Read the model definition and answer for the solid it produces. Units are mm, in the model's axes. A direction names the side the tool comes from. Coordinates: 2 decimals unless noted, no trailing zeros. Write each loop counter-clockwise with the first axis right and the second up, starting at its lowest first coordinate (ties: lowest second). Pieces come first, ordered by that corner, then holes. Notation, with made-up numbers: (73.25, 30.5) -> (131.25, 30.5) arc R3 cw to (131.25, 34.5) -> close; hole circle Ø1 at (39.5, -9.5). An arc over 180 degrees is marked (long way). Return JSON: item names as keys, results as strings.
from build123d import *

# Parameters (mm, degrees)
BOSS_EXTRUDE1_DEPTH = 3
SKETCH2_R           = 3.575
CUT_EXTRUDE1_DEPTH  = 3.95
BOSS_EXTRUDE2_DEPTH = 1.64
SKETCH4_R           = 3.25
CUT_EXTRUDE2_DEPTH  = 4.64


with BuildPart() as part:
    # Sketch1 → Boss-Extrude1 (new body)
    with BuildSketch(Plane(origin=(0, 0, 0), x_dir=(1, 0, 0), z_dir=(0, 1, 0))):
        with BuildLine():
            Line((0, 7), (33, 7))
            ThreePointArc((33, 7), (40, 0), (33, -7))
            Line((33, -7), (0, -7))
            ThreePointArc((0, -7), (-7, 0), (0, 7))
        make_face()
    extrude(amount=BOSS_EXTRUDE1_DEPTH)

    # Sketch2 → Cut-Extrude1 (cut)
    with BuildSketch(Plane.XZ):
        with Locations(Location((0, 0, 0), (0, 0, 270))):
            Circle(SKETCH2_R)
    extrude(amount=-CUT_EXTRUDE1_DEPTH, mode=Mode.SUBTRACT)

    # Sketch3 → Boss-Extrude2 (add)
    with BuildSketch(Plane(origin=(0, 3, 0), x_dir=(1, 0, 0), z_dir=(0, 1, 0))):
        with BuildLine():
            Line((0, -7), (33, -7))
            ThreePointArc((33, -7), (40, 0), (33, 7))
            Line((33, 7), (0, 7))
            ThreePointArc((0, 7), (-7, 0), (0, -7))
        make_face()
        with BuildLine():
            Line((14.43004688, 2.119993993), (2.468524523, 2.816276208))
            ThreePointArc((2.468524523, 2.816276208), (-3.745, 0), (2.468524523, -2.816276208))
            Line((2.468524523, -2.816276208), (14.43004688, -2.119993993))
            ThreePointArc((14.43004688, -2.119993993), (16.545, 0), (14.43004688, 2.119993993))
        make_face(mode=Mode.SUBTRACT)
    extrude(amount=BOSS_EXTRUDE2_DEPTH)

    # Sketch4 → Cut-Extrude2 (cut)
    with BuildSketch(Plane(origin=(0, 4.64, 0), x_dir=(1, 0, 0), z_dir=(0, 1, 0))):
        with Locations(Location((33, 0, 0), (0, 0, 270))):
            Circle(SKETCH4_R)
    extrude(amount=-CUT_EXTRUDE2_DEPTH, mode=Mode.SUBTRACT)


solid = part.part
1. The part is cut by section B-B (y = 3.85). Determine the outline of the cut face in (x, z) (3 decimals), then the cut area to 3 significant figures.
Taken from the geometry:
{"outline": "(0, -7) -> (33, -7) arc R7 ccw to (33, 7) -> (0, 7) arc R7 ccw to start; hole (2.469, -2.816) -> (14.43, -2.12) arc R2.12 ccw to (14.43, 2.12) -> (2.469, 2.816) arc R3.745 ccw (long way) to start; hole circle Ø6.5 at (33, 0)", "area": "478 mm2"}
2. The part is cut by section C-C (x = -0.5). Determine the outline of the cut face in (y, z).
Taken from the geometry:
{"outline": "(0, -6.98) -> (4.64, -6.98) -> (4.64, -3.71) -> (3, -3.71) -> (3, -3.54) -> (0, -3.54) -> close; (0, 3.54) -> (3, 3.54) -> (3, 3.71) -> (4.64, 3.71) -> (4.64, 6.98) -> (0, 6.98) -> close"}
3. A flat-ended cylindrical pin translates along its axis: pin 1 Ø1.5 at (y, z) = (1, 5) entering from -X. Find the tip coordinate at first contact, or state that the pin passes through.
Taken from the geometry:
{"pin 1": "stops at x = -5.56"}
4. Consider L1, parallel to X at y = 2.55, z = 0 (3 decimals); L2, parallel to X at y = 4.25, z = 0 (3 decimals); L3, parallel to Z at x = 0, y = 4.25 (3 decimals). Determine where each line is inside the solid, lowest interval first.
Taken from the geometry:
{"L1": "x = -7 to -3.575, 3.575 to 29.75, 36.25 to 40", "L2": "x = -7 to -3.745, 16.545 to 29.75, 36.25 to 40", "L3": "z = -7 to -3.745, 3.745 to 7"}
5. The part is cut by section D-D (x = 15.5). Determine the outline of the cut face in (y, z), then the cut area to 3 significant figures.
Taken from the geometry:
{"outline": "(0, -7) -> (4.64, -7) -> (4.64, -1.83) -> (3, -1.83) -> (3, 1.83) -> (4.64, 1.83) -> (4.64, 7) -> (0, 7) -> close", "area": "59.0 mm2"}
6. A tool of negligible diameter and unlimited length cuts with its end or side. For faces 5 (the face through (3.545, 1.479, 0.465)), 6 (the face through (16.544, 3.809, 0.047)), from which of +Z, -Z, +X, -X, +Y, -Y can it reach the whole face along a straight path? Write none if from no direction.
Taken from the geometry:
{"face 5": "+Y, -Y", "face 6": "+Y"}
7. The part is cut by section A-A (z = 0). Determine the outline of the cut face in (x, y) (3 decimals), then the cut area to 3 significant figures.
Taken from the geometry:
{"outline": "(-7, 0) -> (-3.575, 0) -> (-3.575, 3) -> (-3.745, 3) -> (-3.745, 4.64) -> (-7, 4.64) -> close; (3.575, 0) -> (29.75, 0) -> (29.75, 4.64) -> (16.545, 4.64) -> (16.545, 3) -> (3.575, 3) -> close; (36.25, 0) -> (40, 0) -> (40, 4.64) -> (36.25, 4.64) -> close", "area": "133 mm2"}
8. For a pull along X with two mould halves and no side action, classify faces 1 (the face through (-7, 2, 0)), 2 (the face through (17, 2, -7)), 3 (the face through (-3.743, 3.809, -0.12)), 4 (the face through (40, 2, 0)) as +X half, -X half, draft (parallel to the pull), parting line (faces both ways), or undercut.
Taken from the geometry:
{"face 1": "-X half", "face 2": "draft", "face 3": "undercut", "face 4": "+X half"}
